```python
from build123d import *

# Parameters (mm, degrees)
SALIENTE_EXTRUIR1_DEPTH      = 3
TALADROAVANZADO1_OUTLINE_R   = 1.2
TALADROAVANZADO1_DEPTH       = 1
TALADROAVANZADO1_DRAFT       = -45
TALADROAVANZADO1_2_OUTLINE_R = 1.2
TALADROAVANZADO1_2_DEPTH     = 1
TALADROAVANZADO1_2_DRAFT     = -45
CORTAR_EXTRUIR1_REACH        = 18.763
CROQUIS3_R                   = 1.243399974
CROQUIS3_R_2                 = 1.156671482
REDONDEO1_R                  = 0.5
REDONDEO2_R                  = 0.5
NGULO_DE_SALIDA1_ANGLE       = 1
REDONDEO3_R                  = 1


# Read off the part's stored shape, not the designer's step: TaladroAvanzado1
with BuildPart() as part:
    # Croquis1 → Saliente-Extruir1 (new, symmetric)
    with BuildSketch(Plane.XY):
        Polygon((-11, 0), (-8, 0), (-8, 3), (8, 3), (8, 0), (11, 0), (16, 0), (16, 3), (11, 3), (11, 6), (-11, 6), (-11, 3), (-16, 3), (-16, 0), align=None)
    extrude(amount=SALIENTE_EXTRUIR1_DEPTH, both=True)


with BuildPart() as taladroavanzado1_tool:
    # TaladroAvanzado1 outline → TaladroAvanzado1 (with draft: the straight prism first)
    with BuildSketch(Plane(origin=(0, 2, 0), x_dir=(1, 0, 0), z_dir=(0, 1, 0))):
        with Locations((13.5, 0)):
            Circle(TALADROAVANZADO1_OUTLINE_R)
    extrude(amount=TALADROAVANZADO1_DEPTH)
    # TaladroAvanzado1: the draft: its side faces are tilted about the plane it starts from
    taladroavanzado1_sides = [taladroavanzado1_tool.faces().sort_by_distance(p)[0] for p in [
        (12.3, 2.5, 0),
    ]]
    draft(taladroavanzado1_sides, Plane(origin=(0, 2, 0), x_dir=(1, 0, 0), z_dir=(0, 1, 0)), TALADROAVANZADO1_DRAFT)


with BuildPart() as part_1:
    add(part.part)

    # TaladroAvanzado1: cut by taladroavanzado1_tool
    add(taladroavanzado1_tool.part, mode=Mode.SUBTRACT)


with BuildPart() as taladroavanzado1_2_tool:
    # TaladroAvanzado1 2 outline → TaladroAvanzado1 2 (with draft: the straight prism first)
    with BuildSketch(Plane(origin=(0, 2, 0), x_dir=(1, 0, 0), z_dir=(0, 1, 0))):
        with Locations((-13.5, 0)):
            Circle(TALADROAVANZADO1_2_OUTLINE_R)
    extrude(amount=TALADROAVANZADO1_2_DEPTH)
    # TaladroAvanzado1 2: the draft: its side faces are tilted about the plane it starts from
    taladroavanzado1_2_sides = [taladroavanzado1_2_tool.faces().sort_by_distance(p)[0] for p in [
        (-14.7, 2.5, 0),
    ]]
    draft(taladroavanzado1_2_sides, Plane(origin=(0, 2, 0), x_dir=(1, 0, 0), z_dir=(0, 1, 0)), TALADROAVANZADO1_2_DRAFT)


with BuildPart() as part_2:
    add(part_1.part)

    # TaladroAvanzado1 2: cut by taladroavanzado1_2_tool
    add(taladroavanzado1_2_tool.part, mode=Mode.SUBTRACT)

    # Croquis3 → Cortar-Extruir1 (cut, up to next)
    with BuildSketch(Plane(origin=(0, 2, 0), x_dir=(1, 0, 0), z_dir=(0, 1, 0)), mode=Mode.PRIVATE) as cortar_extruir1_sk1:
        with Locations(Location((-13.5, 0, 0), (0, 0, 270))):
            Circle(CROQUIS3_R)
    cortar_extruir1_tool1 = extrude(cortar_extruir1_sk1.sketch, amount=-CORTAR_EXTRUIR1_REACH, mode=Mode.PRIVATE) & part_2.part
    # Croquis3 → Cortar-Extruir1 (cut, up to next)
    with BuildSketch(Plane(origin=(0, 2, 0), x_dir=(1, 0, 0), z_dir=(0, 1, 0)), mode=Mode.PRIVATE) as cortar_extruir1_sk2:
        with Locations(Location((13.5, 0, 0), (0, 0, 270))):
            Circle(CROQUIS3_R_2)
    cortar_extruir1_tool2 = extrude(cortar_extruir1_sk2.sketch, amount=-CORTAR_EXTRUIR1_REACH, mode=Mode.PRIVATE) & part_2.part
    add(cortar_extruir1_tool1.solids().sort_by_distance((-13.5, 2, 0))[0], mode=Mode.SUBTRACT)
    add(cortar_extruir1_tool2.solids().sort_by_distance((13.5, 2, 0))[0], mode=Mode.SUBTRACT)

    # Redondeo1
    redondeo1_edges = [part_2.edges().sort_by_distance(p)[0] for p in [
        (8, 3, 0),
        (-8, 3, 0),
    ]]
    fillet(redondeo1_edges, radius=REDONDEO1_R)

    # Redondeo2
    redondeo2_edges = [part_2.edges().sort_by_distance(p)[0] for p in [
        (-11, 6, 0),
        (11, 6, 0),
    ]]
    fillet(redondeo2_edges, radius=REDONDEO2_R)

    # Ángulo de salida1
    ngulo_de_salida1_faces = [part_2.faces().sort_by_distance(p)[0] for p in [
        (0, 3.234018397, 3),
        (0, 3.234018397, -3),
        (16, 1.5, 0),
        (-16, 1.5, 0),
    ]]
    draft(ngulo_de_salida1_faces, Plane(origin=(11, 6, 3), x_dir=(0, 0, 1), z_dir=(0, 1, 0)), NGULO_DE_SALIDA1_ANGLE)

    # Redondeo3
    redondeo3_edges = [part_2.edges().sort_by_distance(p)[0] for p in [
        (-16.078547792, 1.5, -3.078547792),
        (16.078547792, 1.5, -3.078547792),
        (16.078547792, 1.5, 3.078547792),
        (-16.078547792, 1.5, 3.078547792),
    ]]
    fillet(redondeo3_edges, radius=REDONDEO3_R)


solid = part_2.part
```
The listing builds one solid part. Answer for the finished solid, in the listing's coordinates (mm). A direction names the side the tool comes from. Give positions to 0.01 mm unless a question says otherwise; leave off trailing zeros. Order: outer loops, then holes, each group sorted by start corner. A loop starts at its lowest first (then second) coordinate and runs counter-clockwise, first axis right, second up. Notation, with made-up numbers: (-26.75, 13) -> (31.25, 13) arc R7 ccw to (31.25, 26) -> close; hole circle Ø10 at (-36, -16). An arc over 180 degrees is marked (long way). One line per item, written item: value.
1) Flat-ended cylindrical pins translate along their axes: P1, Ø1.2, axis at y = 4, z = 0, coming from the -X side; P2, Ø1.2, axis at y = 4.5, z = 0, coming from the +X side; P3, Ø1, axis at x = -11, y = 2, coming from the +Z side. Find the tip coordinate at first contact, or state that the pin passes through.
Reported:
P1: stops at x = -11
P2: stops at x = 11
P3: stops at z = 3.08
2) Find section C-C, the plane x = -13.5. Determine the outline of the cut face in (y, z), plus the area to 3 significant figures.
Reported:
outline: (0, -3.1) -> (3, -3.05) -> (3, -2.2) -> (2, -1.2) -> (2, -1.24) -> (0, -1.24) -> close; (0, 1.24) -> (2, 1.24) -> (2, 1.2) -> (3, 2.2) -> (3, 3.05) -> (0, 3.1) -> close
area: 10.1 mm^2
3) Determine the mould class of faces 6 (the cylindrical face through (-14.714, 1.014, -0.27)), 7 (the flat face through (-12, 0, 0)), 8 (the cylindrical face through (15.78, 1.52, -2.79)) for opening direction Z: pulls with the +Z half, pulls with the -Z half, needs draft (parallel to the pull), parting line crosses it, or undercut.
Reported:
face 6: undercut
face 7: needs draft
face 8: pulls with the -Z half
4) Find section A-A, the plane x = 13.5. Determine the outline of the cut face in (y, z).
Reported:
outline: (0, -3.1) -> (3, -3.05) -> (3, -2.2) -> (2, -1.2) -> (2, -1.16) -> (0, -1.16) -> close; (0, 1.16) -> (2, 1.16) -> (2, 1.2) -> (3, 2.2) -> (3, 3.05) -> (0, 3.1) -> close
5) Find the intervals of material crossed by line 1 (X direction, y = 1.5, z = 0.75); line 2 (X direction, y = 0.95, z = 0); line 3 (Y direction, x = 7, z = 2.75), in increasing order.
Reported:
line 1: x = -16.08 to -14.49, -12.51 to -8, 8 to 12.62, 14.38 to 16.08
line 2: x = -16.09 to -14.74, -12.26 to -8, 8 to 12.34, 14.66 to 16.09
line 3: y = 3 to 6
6) A tool of negligible diameter and unlimited length cuts with its end or side. For faces 1 (the flat face through (-12, 3, 2)), 2 (the cylindrical face through (-15.79, 1.48, 2.78)), 3 (the cylindrical face through (-15.78, 1.48, -2.79)), 4 (the flat face through (15, 3, -2)), 5 (the flat face through (0, 3, 0)), from which of +Z, -Z, +X, -X, +Y, -Y can it reach the whole face along a straight path? Write none if from no direction.
Reported:
face 1: +Z, -Z, -X, +Y
face 2: +Z, -X, +Y
face 3: -Z, -X, +Y
face 4: +Z, -Z, +X, +Y
face 5: +Z, -Z, -Y
7) Find section B-B, the plane z = 0. Count the separate pieces of the cut face and the enclosed holes in it, plus the area to 3 significant figures.
Reported:
separate pieces: 3
enclosed holes: 0
area: 98.1 mm^2
